Autodesk Inventor part; units mm, degrees
ref_plane "YZ Plane" through (0, 0, 0) normal (1, 0, 0) x (0, 1, 0)
ref_plane "XZ Plane" through (0, 0, 0) normal (0, 1, 0) x (-1, 0, 0)
ref_plane "XY Plane" through (0, 0, 0) normal (0, 0, 1) x (1, 0, 0)
sketch "Эскиз1" plane through (0, 0, 0) normal (0, 0, 1) x (1, 0, 0)
  line L0 (0, -7.62) -> (65.71, -7.62)
  line L1 (65.71, -7.62) -> (65.71, 29.2)
  line L2 (65.71, 29.2) -> (0, 29.2)
  line L3 (0, 29.2) -> (0, -7.62)
  circle A0 centre (3.81, 15.24) radius 0.8
  circle A1 centre (3.81, 20.24) radius 0.8
  circle A2 centre (3.81, 2.54) radius 0.8
  circle A3 centre (3.81, 7.54) radius 0.8
  circle A4 centre (51.94, 3.18) radius 0.5
  circle A5 centre (54.48, 3.18) radius 0.5
  circle A6 centre (2.54, 26.67) radius 1.6
  circle A7 centre (2.54, -5.08) radius 1.6
  circle A8 centre (63.5, -5.08) radius 1.6
  circle A9 centre (63.5, 26.67) radius 1.6
extrude "untitled.brdКонтур" add sketch "Эскиз1" along normal blind 1.6
properties part number "untitled.brdКонтур"
CAD build for the part. Positions are in the model's coordinates, mm. Give positions to 0.01 mm unless a question says otherwise; leave off trailing zeros. Loops run counter-clockwise (first coordinate to the right, second up) from the corner with the lowest first, then second, coordinate; pieces in that order, holes last. Notation, with made-up numbers: M 41,48.5 L 55,48.5 A15 cw 55,60.5 Z; hole C -30.75,22 d2. An arc over 180 degrees is marked long. Answer in a Markdown table with one row per item. Add a question column.
Item 1: Band-saw the part on B-B on z = 0.9. Give the number of separate pieces and of enclosed holes in the cut face, then the cut area to 3 significant figures.
Item 2: Band-saw the part on C-C on y = 20.24. Give the cut face in (x, z).
Item 3: Band-saw the part on A-A on x = 63.5. Give the cut face in (y, z).
Item 4: Probe probe 1 along X at (y, z) = (-5, 0.45); probe 2 along Y at (x, z) = (51.94, 0.6). List the from-to ranges inside material, lowest first.
Item 5: Band-saw the part on D-D on y = -5.08. Give the cut face in (x, z).
Item 6: Drop a flat-ended pin along its axis: P1, Ø3.5, axis at x = 2.54, y = -5.08, coming from the +Z side. Give the stop position or say it passes through.
Item 7: Mould opens along Y. For faces 1 (the face through (32, 11, 1.6)), 2 (the face through (32, -7.62, 1)), 3 (the face through (4.18, 20.95, 0.79)), 4 (the face through (2.332, -6.666, 0.789)) say: +Y half, -Y half, draft (parallel to the pull), parting line (faces both ways), or undercut.
Reply:
| question | item | result |
|---|---|---|
| 1 | separate pieces | 1 |
| 1 | enclosed holes | 10 |
| 1 | area | 2,380 mm^2 |
| 2 | outline | M 0,0 L 3.01,0 L 3.01,1.6 L 0,1.6 Z; M 4.61,0 L 65.71,0 L 65.71,1.6 L 4.61,1.6 Z |
| 3 | outline | M -7.62,0 L -6.68,0 L -6.68,1.6 L -7.62,1.6 Z; M -3.48,0 L 25.07,0 L 25.07,1.6 L -3.48,1.6 Z; M 28.27,0 L 29.2,0 L 29.2,1.6 L 28.27,1.6 Z |
| 4 | probe 1 | x = 0 to 0.94, 4.14 to 61.9, 65.1 to 65.71 |
| 4 | probe 2 | y = -7.62 to 2.68, 3.68 to 29.2 |
| 5 | outline | M 0,0 L 0.94,0 L 0.94,1.6 L 0,1.6 Z; M 4.14,0 L 61.9,0 L 61.9,1.6 L 4.14,1.6 Z; M 65.1,0 L 65.71,0 L 65.71,1.6 L 65.1,1.6 Z |
| 6 | P1 | stops at z = 1.6 |
| 7 | face 1 | draft |
| 7 | face 2 | -Y half |
| 7 | face 3 | undercut |
| 7 | face 4 | undercut |
